The figure shows three views and two pictorial views of one solid part (mm, origin at its lowest corner). Answer the questions. A direction names the side the tool comes from. Give positions to 0.01 mm unless a question says otherwise; leave off trailing zeros. Loops run counter-clockwise (first coordinate to the right, second up) from the corner with the lowest first, then second, coordinate; pieces in that order, holes last. Notation, with made-up numbers: (78, -13) -> (116, -13) arc R6 cw to (116, -3) -> close; hole circle Ø1 at (63.5, 53.5). An arc over 180 degrees is marked (long way). Answer as CSV lines item,"result". Start each with the question number.
1. A flat-ended cylindrical pin translates along its axis: pin 1 Ø3 at (x, z) = (21.9, 6.1) entering from -Y. Find the tip coordinate at first contact, or state that the pin passes through.
2. Determine the mould class of the marked faces 1, 2 and 3 for opening direction Z: +Z half, -Z half, draft (parallel to the pull), parting line (faces both ways), or undercut.
3. Find section A-A, the plane z = 9.5. Give the vertices of the cut face in (x, y) (3 decimals).
4. Find section C-C, the plane z = 7.5. Give the vertices of the cut face in (x, y) (1 decimal).
5. Find section D-D, the plane x = 22.5. Give the vertices of the cut face in (y, z).
6. Find the intervals of material crossed by line 1 along Y through (x, z) = (17.75, 2); line 2 along X through (y, z) = (7.5, 5.5) (1 decimal); line 3 along X through (y, z) = (8.25, 4.5) (1 decimal), in increasing order.
7. A tool of negligible diameter and unlimited length cuts with its end or side. For the marked faces 4 and 5, from which of +Z, -Z, +X, -X, +Y, -Y can it reach the whole face along a straight path? Write none if from no direction.
8. Find section B-B, the plane x = 8.25. Give the vertices of the cut face in (y, z).
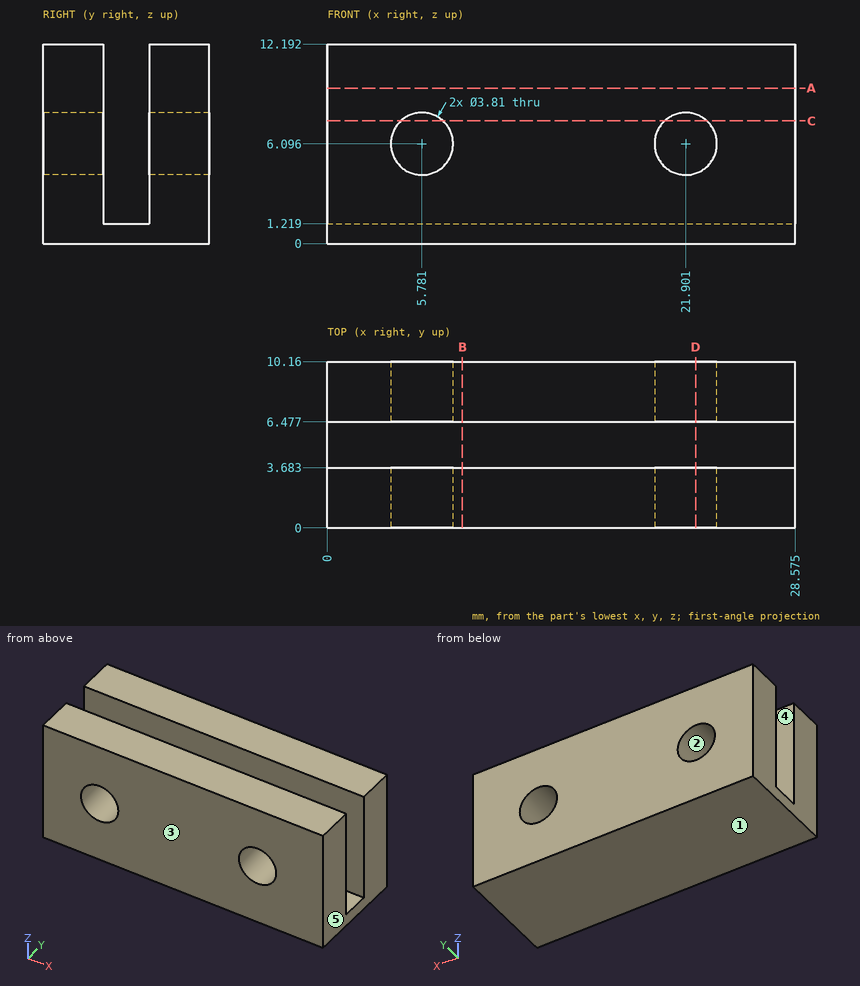
Resolved:
1,pin 1,"passes through"
2,face 1,"-Z half"
2,face 2,"undercut"
2,face 3,"draft"
3,outline,"(0, 0) -> (28.575, 0) -> (28.575, 3.683) -> (0, 3.683) -> close; (0, 6.477) -> (28.575, 6.477) -> (28.575, 10.16) -> (0, 10.16) -> close"
4,outline,"(0, 0) -> (4.5, 0) -> (4.5, 3.7) -> (0, 3.7) -> close; (0, 6.5) -> (4.5, 6.5) -> (4.5, 10.2) -> (0, 10.2) -> close; (7.1, 0) -> (20.6, 0) -> (20.6, 3.7) -> (7.1, 3.7) -> close; (7.1, 6.5) -> (20.6, 6.5) -> (20.6, 10.2) -> (7.1, 10.2) -> close; (23.2, 0) -> (28.6, 0) -> (28.6, 3.7) -> (23.2, 3.7) -> close; (23.2, 6.5) -> (28.6, 6.5) -> (28.6, 10.2) -> (23.2, 10.2) -> close"
5,outline,"(0, 0) -> (10.16, 0) -> (10.16, 4.29) -> (6.48, 4.29) -> (6.48, 1.22) -> (3.68, 1.22) -> (3.68, 4.29) -> (0, 4.29) -> close; (0, 7.9) -> (3.68, 7.9) -> (3.68, 12.19) -> (0, 12.19) -> close; (6.48, 7.9) -> (10.16, 7.9) -> (10.16, 12.19) -> (6.48, 12.19) -> close"
6,line 1,"y = 0 to 3.68, 6.48 to 10.16"
6,line 2,"x = 0 to 4, 7.6 to 20.1, 23.7 to 28.6"
6,line 3,"x = 0 to 4.7, 6.8 to 20.9, 22.9 to 28.6"
7,face 4,"+Z, +X, -X"
7,face 5,"+Z, -Z, +X, +Y, -Y"
8,outline,"(0, 0) -> (10.16, 0) -> (10.16, 12.19) -> (6.48, 12.19) -> (6.48, 1.22) -> (3.68, 1.22) -> (3.68, 12.19) -> (0, 12.19) -> close"
